Here's how the part is built. I have some questions about the finished solid (model axes, mm). Round coordinates to 2 decimals unless told otherwise and drop trailing zeros. Write each loop counter-clockwise with the first axis right and the second up, starting at its lowest first coordinate (ties: lowest second). Pieces come first, ordered by that corner, then holes. Notation, with made-up numbers: (14, 19.25) -> (22, 19.25) arc R22 ccw to (22, 58.25) -> close; hole circle Ø5 at (7, -2.5). An arc over 180 degrees is marked (long way). Answer as CSV lines item,"result".
```python
from build123d import *

# Parameters (mm, degrees)
F1_DEPTH      = 8.89
F3_DEPTH      = 4.9276
F3_DEPTH_BACK = 2.54
F7_DEPTH      = 13.6535
F8_W          = 330.2
F8_H          = 330.2
F9_DEPTH      = 8.9916
F13_DEPTH     = 25.4
F15_DEPTH     = 8.9926
F16_W         = 7.7724
F16_H         = 50.8
F16_W_2       = 1.4224
F16_H_2       = 44.069
F17_DEPTH     = 8.9926


with BuildPart() as f1:
    # F0 (on Top) → F1 (new body)
    with BuildSketch(Plane.XY):
        with BuildLine():
            Line((67.3940027121, -114.3), (111.125, -114.3))
            ThreePointArc((111.125, -114.3), (113.3700640303, -113.3700640303), (114.3, -111.125))
            Line((114.3, -111.125), (114.3, 85.344))
            ThreePointArc((114.3, 85.344), (115.2299359697, 87.5890640303), (117.475, 88.519))
            Line((117.475, 88.519), (123.825, 88.519))
            ThreePointArc((123.825, 88.519), (126.0700640303, 89.4489359697), (127, 91.694))
            Line((127, 91.694), (127, 111.125))
            ThreePointArc((127, 111.125), (126.0700640303, 113.3700640303), (123.825, 114.3))
            Line((123.825, 114.3), (114.3, 114.3))
            Line((114.3, 114.3), (-111.125, 114.3))
            ThreePointArc((-111.125, 114.3), (-113.3700640303, 113.3700640303), (-114.3, 111.125))
            Line((-114.3, 111.125), (-114.3, -111.125))
            ThreePointArc((-114.3, -111.125), (-113.3700640303, -113.3700640303), (-111.125, -114.3))
            Line((-111.125, -114.3), (-67.3940027121, -114.3))
            ThreePointArc((-67.3940027121, -114.3), (-66.0408699293, -114.6027784431), (-64.9458155322, -115.4533658758))
            ThreePointArc((-64.9458155322, -115.4533658758), (0, -146.05), (64.9458155322, -115.4533658758))
            ThreePointArc((64.9458155322, -115.4533658758), (66.0408699293, -114.6027784431), (67.3940027121, -114.3))
        make_face()
    extrude(amount=F1_DEPTH)

    # F2 (on face) → F3 (join, two sides)
    with BuildSketch(Plane.YZ.offset(114.3)) as f3_sk:
        Polygon((50.8, -3.175), (66.675, -3.175), (69.85, -4.7625), (69.85, -1.9226936686), (67.2746126628, -0.635), (51.3996126628, -0.635), (50.1296126628, 0), (44.45, 0), align=None)
        Polygon((44.45, 2.8398063314), (44.45, 0), (50.1296126628, 0), align=None)
    extrude(amount=F3_DEPTH)
    extrude(f3_sk.sketch, amount=-F3_DEPTH_BACK)


with BuildPart() as f4_1:
    # F4: copy of F1
    add(f1.part.moved(Location((0, -114.3, 0))))


with BuildPart() as f1_1:
    add(f1.part)

    add(f4_1.part)  # F5 merges F4_1
    # F5: F1, F4_1 across plane
    add(f1.part.mirror(Plane.YZ))
    add(f4_1.part.mirror(Plane.YZ))

    # F6 (on face) → F7 (cut, through all)
    with BuildSketch(Plane.XY.offset(8.89)):
        with BuildLine():
            Line((33.2011497354, -114.3), (-33.2011497354, -114.3))
            ThreePointArc((-33.2011497354, -114.3), (-37.5757853229, -117.1799565804), (-36.6596028328, -122.33671875))
            ThreePointArc((-36.6596028328, -122.33671875), (0, -138.1125), (36.6596028328, -122.33671875))
            ThreePointArc((36.6596028328, -122.33671875), (37.5757853229, -117.1799565804), (33.2011497354, -114.3))
        make_face()
    extrude(amount=-F7_DEPTH, mode=Mode.SUBTRACT)


with BuildPart() as f9:
    # F8 (on Top) → F9 (new body)
    with BuildSketch(Plane.XY):
        Rectangle(F8_W, F8_H)
        with BuildLine():
            ThreePointArc((-114.3, 111.125), (-113.3700640303, 113.3700640303), (-111.125, 114.3))
            Line((-111.125, 114.3), (123.825, 114.3))
            ThreePointArc((123.825, 114.3), (126.0700640303, 113.3700640303), (127, 111.125))
            Line((127, 111.125), (127, 91.694))
            ThreePointArc((127, 91.694), (126.0700640303, 89.4489359697), (123.825, 88.519))
            Line((123.825, 88.519), (117.475, 88.519))
            ThreePointArc((117.475, 88.519), (115.2299359697, 87.5890640303), (114.3, 85.344))
            Line((114.3, 85.344), (114.3, 69.85))
            Line((114.3, 69.85), (119.2276, 69.85))
            Line((119.2276, 69.85), (119.2276, 67.2746126628))
            Line((119.2276, 67.2746126628), (119.2276, 51.3996126628))
            Line((119.2276, 51.3996126628), (119.2276, 44.45))
            Line((119.2276, 44.45), (114.3, 44.45))
            Line((114.3, 44.45), (114.3, -44.45))
            Line((114.3, -44.45), (119.2276, -44.45))
            Line((119.2276, -44.45), (119.2276, -47.0253873372))
            Line((119.2276, -47.0253873372), (119.2276, -62.9003873372))
            Line((119.2276, -62.9003873372), (119.2276, -69.85))
            Line((119.2276, -69.85), (114.3, -69.85))
            Line((114.3, -69.85), (114.3, -111.125))
            ThreePointArc((114.3, -111.125), (113.3700640303, -113.3700640303), (111.125, -114.3))
            Line((111.125, -114.3), (67.3940027121, -114.3))
            ThreePointArc((67.3940027121, -114.3), (66.0408699293, -114.6027784431), (64.9458155322, -115.4533658758))
            ThreePointArc((64.9458155322, -115.4533658758), (0, -146.05), (-64.9458155322, -115.4533658758))
            ThreePointArc((-64.9458155322, -115.4533658758), (-66.0408699293, -114.6027784431), (-67.3940027121, -114.3))
            Line((-67.3940027121, -114.3), (-111.125, -114.3))
            ThreePointArc((-111.125, -114.3), (-113.3700640303, -113.3700640303), (-114.3, -111.125))
            Line((-114.3, -111.125), (-114.3, -69.85))
            Line((-114.3, -69.85), (-119.2276, -69.85))
            Line((-119.2276, -69.85), (-119.2276, -62.9003873372))
            Line((-119.2276, -62.9003873372), (-119.2276, -47.0253873372))
            Line((-119.2276, -47.0253873372), (-119.2276, -44.45))
            Line((-119.2276, -44.45), (-114.3, -44.45))
            Line((-114.3, -44.45), (-114.3, 44.45))
            Line((-114.3, 44.45), (-119.2276, 44.45))
            Line((-119.2276, 44.45), (-119.2276, 51.3996126628))
            Line((-119.2276, 51.3996126628), (-119.2276, 67.2746126628))
            Line((-119.2276, 67.2746126628), (-119.2276, 69.85))
            Line((-119.2276, 69.85), (-114.3, 69.85))
            Line((-114.3, 69.85), (-114.3, 111.125))
        make_face(mode=Mode.SUBTRACT)
    extrude(amount=F9_DEPTH)

    # F11 (on face) → F13 (cut)
    with BuildSketch(Plane.XY.offset(8.9916)):
        with BuildLine():
            ThreePointArc((123.825, 114.3), (124.3749261314, 114.2520123521), (124.9082288539, 114.1095))
            ThreePointArc((124.9082288539, 114.1095), (126.4249881357, 115.2717248577), (127, 117.094))
            Line((127, 117.094), (127, 136.525))
            ThreePointArc((127, 136.525), (126.0700640303, 138.7700640303), (123.825, 139.7))
            Line((123.825, 139.7), (-111.125, 139.7))
            ThreePointArc((-111.125, 139.7), (-113.3700640303, 138.7700640303), (-114.3, 136.525))
            Line((-114.3, 136.525), (-114.3, 111.125))
            ThreePointArc((-114.3, 111.125), (-113.3700640303, 113.3700640303), (-111.125, 114.3))
            Line((-111.125, 114.3), (123.825, 114.3))
        make_face()
        Polygon((-114.3, 69.85), (-114.3, 95.25), (-119.2276, 95.25), (-119.2276, 92.6746126628), (-119.2276, 76.7996126628), (-119.2276, 69.85), align=None)
        Polygon((-114.3, -44.45), (-114.3, -19.05), (-119.2276, -19.05), (-119.2276, -21.6253873372), (-119.2276, -37.5003873372), (-119.2276, -44.45), align=None)
        Polygon((119.2276, -19.05), (114.3, -19.05), (114.3, -44.45), (119.2276, -44.45), (119.2276, -37.5003873372), (119.2276, -21.6253873372), align=None)
        with BuildLine():
            ThreePointArc((117.475, 88.519), (115.2299359697, 87.5890640303), (114.3, 85.344))
            Line((114.3, 85.344), (114.3, 69.85))
            Line((114.3, 69.85), (119.2276, 69.85))
            Line((119.2276, 69.85), (119.2276, 76.7996126628))
            Line((119.2276, 76.7996126628), (119.2276, 88.519))
            Line((119.2276, 88.519), (117.475, 88.519))
        make_face()
    extrude(amount=-F13_DEPTH, mode=Mode.SUBTRACT)

    # F14 (on face) → F15 (cut, through all)
    with BuildSketch(Plane.XY.offset(8.9916)):
        with BuildLine():
            Line((127, 111.125), (127, 117.094))
            ThreePointArc((127, 117.094), (126.4249881357, 115.2717248577), (124.9082288539, 114.1095))
            ThreePointArc((124.9082288539, 114.1095), (126.4249881357, 112.9472751423), (127, 111.125))
        make_face()
    extrude(amount=-F15_DEPTH, mode=Mode.SUBTRACT)

    # F16 (on face) → F17 (cut, through all)
    with BuildSketch(Plane.XY.offset(8.9916)):
        with Locations((-123.1138, 69.85)):
            Rectangle(F16_W, F16_H)
        with Locations((-123.1138, -44.45)):
            Rectangle(F16_W, F16_H)
        with Locations((123.1138, -44.45)):
            Rectangle(F16_W, F16_H)
        with Locations((119.9388, 66.4845)):
            Rectangle(F16_W_2, F16_H_2)
    extrude(amount=-F17_DEPTH, mode=Mode.SUBTRACT)


with BuildPart() as f1_2:
    # F10: moved
    add(f1_1.part.moved(Location((0, 25.4, 0))))


solid = f9.part
```
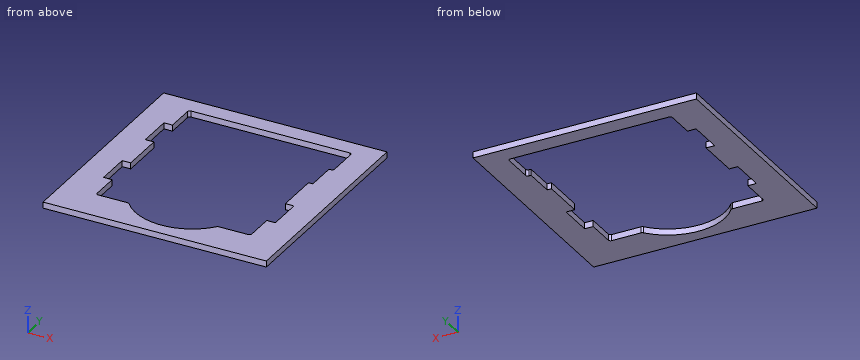
1. If I drill on line 1 (Y direction, x = -118.5, z = 0.5); line 2 (X direction, y = 104, z = 3.75); line 3 (Y direction, x = -100, z = 8), over which ranges is the centre line in solid material (lowest first)?
Numbers:
line 1,"y = -165.1 to -69.85, -19.05 to 44.45, 95.25 to 165.1"
line 2,"x = -165.1 to -114.3, 127 to 165.1"
line 3,"y = -165.1 to -114.3, 139.7 to 165.1"
2. Suppose I cut it at A-A on x = 82.5. Please give me the cut outline in (y, z), and give its area (3 significant figures).
Numbers:
outline,"(-165.1, 0) -> (-114.3, 0) -> (-114.3, 8.99) -> (-165.1, 8.99) -> close; (139.7, 0) -> (165.1, 0) -> (165.1, 8.99) -> (139.7, 8.99) -> close"
area,"685 mm^2"
3. Suppose I cut it at B-B on y = -76.5. Please give me the cut outline in (x, z), and give its area (3 significant figures).
Numbers:
outline,"(-165.1, 0) -> (-114.3, 0) -> (-114.3, 8.99) -> (-165.1, 8.99) -> close; (114.3, 0) -> (165.1, 0) -> (165.1, 8.99) -> (114.3, 8.99) -> close"
area,"914 mm^2"
